```python
from build123d import *

# Parameters (mm, degrees)
BOSS_EXTRUDE2_DEPTH = 1117.6
SKETCH3_R           = 10
CUT_EXTRUDE1_DEPTH  = 1117.6


with BuildPart() as part:
    # Sketch2 → Boss-Extrude2 (new body)
    with BuildSketch(Plane.XY):
        with BuildLine():
            Line((0, -50.8), (-635, -50.8))
            ThreePointArc((-635, -50.8), (-685.8, 0), (-635, 50.8))
            Line((-635, 50.8), (0, 50.8))
            ThreePointArc((0, 50.8), (50.8, 0), (0, -50.8))
        make_face()
    extrude(amount=BOSS_EXTRUDE2_DEPTH)

    # Sketch3 → Cut-Extrude1 (cut)
    with BuildSketch(Plane.XY.offset(1117.6)):
        with Locations((-635, 0)):
            Circle(SKETCH3_R)
        with BuildLine():
            Line((0, -43.104643513), (-506.395864425, -43.104643513))
            ThreePointArc((-506.395864425, -43.104643513), (-549.500507938, 0), (-506.395864425, 43.104643513))
            Line((-506.395864425, 43.104643513), (0, 43.104643513))
            ThreePointArc((0, 43.104643513), (43.104643513, 0), (0, -43.104643513))
        make_face()
    extrude(amount=-CUT_EXTRUDE1_DEPTH, mode=Mode.SUBTRACT)


solid = part.part
```
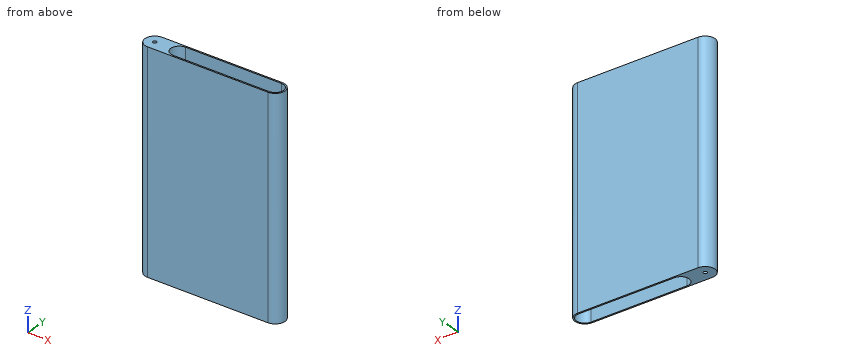
Design review of the part built by this model. Coordinates are the model's own, in mm. Round coordinates to 2 decimals unless told otherwise and drop trailing zeros. Order: outer loops, then holes, each group sorted by start corner. A loop starts at its lowest first (then second) coordinate and runs counter-clockwise, first axis right, second up. Notation, with made-up numbers: (26, 18) - (31, 18) arc R18 cw to (31, 32) - close; hole circle Ø10 at (23, 41.25). An arc over 180 degrees is marked (long way). Return JSON: item names as keys, results as strings.
Q1. Wall thickness on L1, parallel to Y at x = -94.5, z = 586; L2, parallel to Y at x = -635, z = 277.5; L3, parallel to X at y = 33.5, z = 652: over which ranges is each line inside the solid? List them lowest first. Write a range as [from, to].
Computed values:
{"L1": "y = [-50.8, -43.1], [43.1, 50.8]", "L2": "y = [-50.8, -10], [10, 50.8]", "L3": "x = [-673.19, -533.52], [27.12, 38.19]"}
Q2. Consider section C-C on x = -518. Write out the cut boundary in (y, z).
Computed values:
{"outline": "(-50.8, 0) - (-41.51, 0) - (-41.51, 1117.6) - (-50.8, 1117.6) - close; (41.51, 0) - (50.8, 0) - (50.8, 1117.6) - (41.51, 1117.6) - close"}
Q3. Consider section B-B on z = 397.5. Write out the cut boundary in (x, y).
Computed values:
{"outline": "(-635, -50.8) - (0, -50.8) arc R50.8 ccw to (0, 50.8) - (-635, 50.8) arc R50.8 ccw to start; hole circle Ø20 at (-635, 0); hole (-506.4, -43.1) - (0, -43.1) arc R43.1 ccw to (0, 43.1) - (-506.4, 43.1) arc R43.1 ccw to start"}
Q4. Consider section A-A on x = -65.5. Write out the cut boundary in (y, z), plus the area to 3 significant figures.
Computed values:
{"outline": "(-50.8, 0) - (-43.1, 0) - (-43.1, 1117.6) - (-50.8, 1117.6) - close; (43.1, 0) - (50.8, 0) - (50.8, 1117.6) - (43.1, 1117.6) - close", "area": "17,200 mm2"}
Q5. For pin 1 Ø1.5 at (y, z) = (38, 226) entering from -X; pin 2 Ø3 at (y, z) = (-2.5, 608) entering from -X; pin 3 Ø18 at (x, y) = (-635, 0) entering from -Z, all flat-tipped, find the tip position at first contact; note any pin that passes through.
Computed values:
{"pin 1": "stops at x = -669.54", "pin 2": "stops at x = -685.79", "pin 3": "passes through"}
